The model under review builds one solid part; all positions refer to its coordinate system, in mm. A direction names the side the tool comes from. Give positions to 0.01 mm unless a question says otherwise; leave off trailing zeros. Write each loop counter-clockwise with the first axis right and the second up, starting at its lowest first coordinate (ties: lowest second). Pieces come first, ordered by that corner, then holes. Notation, with made-up numbers: (-29, -12) - (-25, -12) arc R31 cw to (-25, 24) - close; hole circle Ø11 at (59, -27.75). An arc over 180 degrees is marked (long way). Write item = value, one per line.
```python
from build123d import *

# Parameters (mm, degrees)
SKETCH_1_R             = 35
SM_BASE_FLANGE_1_DEPTH = 30
FILLET_1_R             = 20
FILLET_2_R             = 13
FILLET_3_R             = 5
HOLE_WIZARD_M12_1_D    = 10.2
CHAMFER_1_SIZE         = 5
CHAMFER_2_SIZE         = 1


# Sheet-metal steps are written as plain solids
with BuildPart() as part:
    # Sketch 1 → 基体-法兰1 (new body)
    with BuildSketch(Plane.XY):
        with BuildLine():
            Line((-303, 50), (-303, 27))
            Line((-303, 27), (-90, 27))
            Line((-90, 27), (-90, -82))
            Line((-90, -82), (-78, -82))
            Line((-78, -82), (-78, -94))
            Line((-78, -94), (37, -94))
            Line((37, -94), (61.618237028, -20.692821595))
            ThreePointArc((61.618237028, -20.692821595), (52.77325745, 37.947111855), (0, 65))
            Line((0, 65), (-253, 65))
            Line((-253, 65), (-303, 50))
        make_face()
        Circle(SKETCH_1_R, mode=Mode.SUBTRACT)
    extrude(amount=-SM_BASE_FLANGE_1_DEPTH)

    # 圆角1
    fillet_1_edges = [part.edges().sort_by_distance(p)[0] for p in [
        (-253, 65, -15),
    ]]
    fillet(fillet_1_edges, radius=FILLET_1_R)

    # 圆角2
    fillet_2_edges = [part.edges().sort_by_distance(p)[0] for p in [
        (-90, 27, -15),
    ]]
    fillet(fillet_2_edges, radius=FILLET_2_R)

    # 圆角3
    fillet_3_edges = [part.edges().sort_by_distance(p)[0] for p in [
        (-78, -82, -15),
    ]]
    fillet(fillet_3_edges, radius=FILLET_3_R)

    # M12 螺纹孔1 (through all)
    with Locations(Plane.XY):
        with Locations((-64.951905284, 37.5)):
            Hole(HOLE_WIZARD_M12_1_D / 2)

    # 倒角1
    chamfer_1_edges = [part.edges().sort_by_distance(p)[0] for p in [
        (-203, 27, 0),
        (-90, -82, -15),
        (-203, 27, -30),
        (-90, -34, 0),
        (-90, -34, -30),
        (-93.807611845, 23.192388155, 0),
        (-93.807611845, 23.192388155, -30),
    ]]
    chamfer(chamfer_1_edges, length=CHAMFER_1_SIZE)

    # 倒角2
    chamfer_2_edges = [part.edges().sort_by_distance(p)[0] for p in [
        (-35, 0, -30),
        (-35, 0, 0),
    ]]
    chamfer(chamfer_2_edges, length=CHAMFER_2_SIZE)


solid = part.part
```
1. For line 1 (Y direction, x = 0, z = -23); line 2 (X direction, y = 1, z = -10); line 3 (X direction, y = -22, z = -24), list the stretches that pass through material, from the lowest coordinate up. Write a range as from..to.
Findings below:
line_1 = -94..-35, 35..65
line_2 = -90..-34.99, 34.99..64.99
line_3 = -90..-27.22, 27.22..61.18
2. Take a section at D-D on y = -58. Give the boundary of the cut face in (x, z), and give its area (3 significant figures).
Findings below:
outline = (-90, -25) - (-85, -30) - (49.09, -30) - (49.09, 0) - (-85, 0) - (-90, -5) - close
area = 4,150 mm²
3. Draft analysis for pull direction X (two halves, no side actions). For faces 3 (the cylindrical face through (-69.816, 39.032, -15.21)), 4 (the flat face through (-81, 4, 0)), 5 (the conical face through (-92.53, 24.71, -26.98)), state which applies: +X half, -X half, draft (parallel to the pull), parting line (faces both ways), or undercut.
Findings below:
face_3 = undercut
face_4 = draft
face_5 = -X half
4. Take a section at C-C on x = -187.5. Give the boundary of the cut face in (y, z).
Findings below:
outline = (27, -25) - (32, -30) - (65, -30) - (65, 0) - (32, 0) - (27, -5) - close
5. Take a section at A-A on y = 0. Give the boundary of the cut face in (x, z).
Findings below:
outline = (-90, -25) - (-85, -30) - (-36, -30) - (-35, -29) - (-35, -1) - (-36, 0) - (-85, 0) - (-90, -5) - close; (35, -29) - (36, -30) - (65, -30) - (65, 0) - (36, 0) - (35, -1) - close
6. Machinability: for faces 1 (the flat face through (-81, 4, -30)), 2 (the flat face through (-204, 27, -15)), which of the approach directions +Z, -Z, +X, -X, +Y, -Y give a long, thin tool a straight path to every point of the face, cutting with its end or side? Answer none if there is none.
Findings below:
face_1 = -Z, +X, -X, +Y, -Y
face_2 = +Z, -Z, -X, -Y
7. Take a section at B-B on z = -11.5. Give the boundary of the cut face in (x, y), and give its area (3 significant figures).
Findings below:
outline = (-303, 27) - (-103, 27) arc R13 cw to (-90, 14) - (-90, -77) - (-85, -82) - (-83, -82) arc R5 cw to (-78, -87) - (-78, -94) - (37, -94) - (61.62, -20.69) arc R65 ccw to (0, 65) - (-250.06, 65) arc R20 ccw to (-255.81, 64.16) - (-303, 50) - close; hole circle Ø10.2 at (-64.95, 37.5); hole circle Ø70 at (0, 0)
area = 26,200 mm²
8. Insertion check: P1, Ø10, axis at y = -49.5, z = -10, coming from the -X side; P2, Ø1.5, axis at y = -43, z = -3, coming from the -X side; P3, Ø6, axis at x = -228, z = -16, coming from the -Y side. Each pin has a flat end and moves straight along its axis. Give the tip position at first contact, or say it passes through.
Findings below:
P1 = -90
P2 = -88.75
P3 = 27
